Answer from the drawing. Dimensions are ordinates in mm from the lowest x, y and z of the part. A direction names the side the tool comes from. Give positions to 0.01 mm unless a question says otherwise; leave off trailing zeros. Loops run counter-clockwise (first coordinate to the right, second up) from the corner with the lowest first, then second, coordinate; pieces in that order, holes last. Notation, with made-up numbers: (15.5, -5) - (56.5, -5) arc R27 cw to (56.5, 18) - close; hole circle Ø4 at (36, -1). An arc over 180 degrees is marked (long way). Answer as CSV lines item,"result". Start each with the question number.
1) Find the intervals of material crossed by line 1 along X through (y, z) = (9, 35) (1 decimal); line 2 along Y through (x, z) = (44, 141); line 3 along X through (y, z) = (18, 95) (1 decimal), in increasing order.
2) For the marked faces 1 and 2, determine the directions among +Z, -Z, +X, -X, +Y, -Y from which every point of the face is accessible in a straight line to the end or side of a thin tool.
3) For a pull along X with two mould halves and no side action, classify the marked faces 3, 4 and 5 as pulls with the +X half, pulls with the -X half, needs draft (parallel to the pull), parting line crosses it, or undercut.
4) Flat-ended cylindrical pins translate along their axes: pin 1 (1 mm diameter, centred on y = 16, z = 100, fed in from -X); pin 2 (10 mm diameter, centred on y = 9, z = 82.5, fed in from +X); pin 3 (23 mm diameter, centred on x = 43, z = 124, fed in from -Y) (1 decimal); pin 4 (3.5 mm diameter, centred on y = 16, z = 98, fed in from +X) (1 decimal). Find the tip coordinate at first contact, or state that the pin passes through.
5) A cutting plane is placed at C-C (z = 120.5). Determine the outline of the cut face in (x, y).
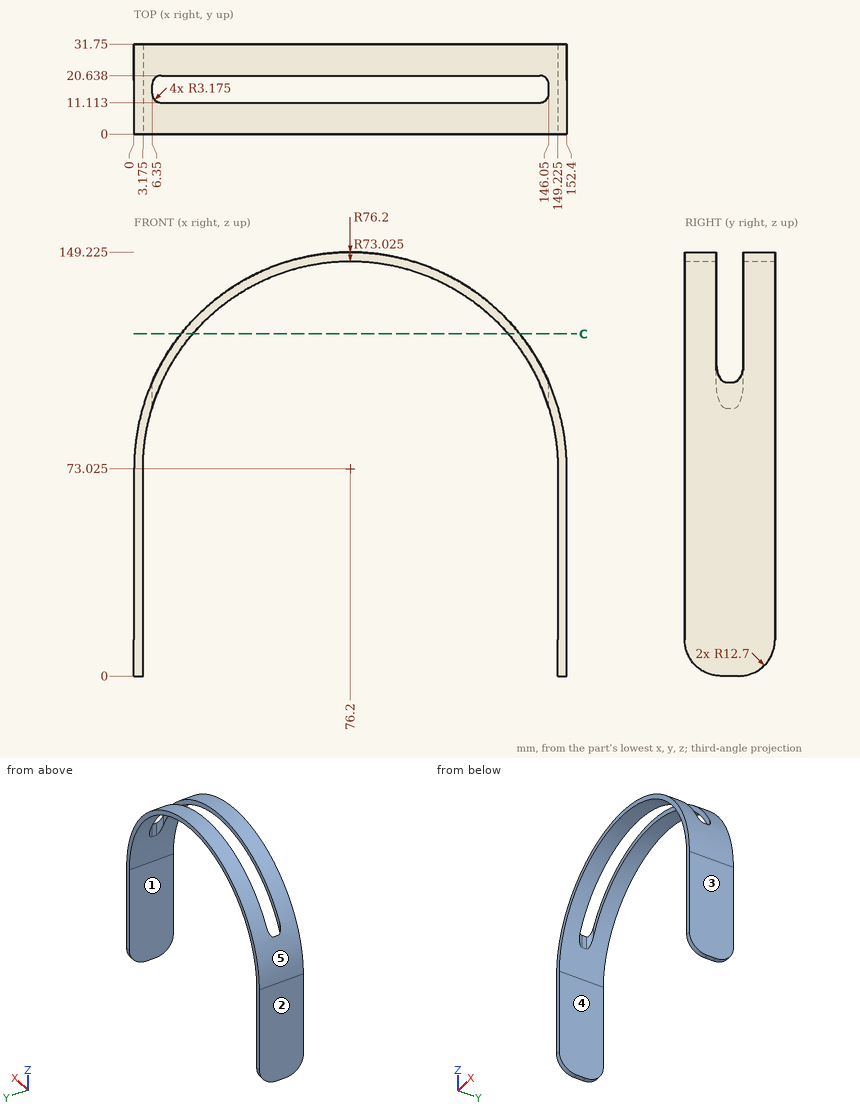
Ans:
1,line 1,"0 to 3.2, 149.2 to 152.4"
1,line 2,"0 to 11.11, 20.64 to 31.75"
1,line 3,"3.2 to 6.4, 146 to 149.2"
2,face 1,"-Z, +Y, -Y"
2,face 2,"+Z, -Z, -X, +Y, -Y"
3,face 3,"pulls with the +X half"
3,face 4,"undercut"
3,face 5,"parting line crosses it"
4,pin 1,"x = 4.75"
4,pin 2,"x = 152.27"
4,pin 3,"through"
4,pin 4,"x = 148.8"
5,outline,"(16.6, 0) - (20.71, 0) - (20.71, 11.11) - (16.6, 11.11) - close; (16.6, 20.64) - (20.71, 20.64) - (20.71, 31.75) - (16.6, 31.75) - close; (131.69, 0) - (135.8, 0) - (135.8, 11.11) - (131.69, 11.11) - close; (131.69, 20.64) - (135.8, 20.64) - (135.8, 31.75) - (131.69, 31.75) - close"
